Source: three-view drawing plus pictorial views. Frame: mm from the lowest corner of the part. A direction names the side the tool comes from. Coordinates: 2 decimals unless noted, no trailing zeros. Order: outer loops, then holes, each group sorted by start corner. A loop starts at its lowest first (then second) coordinate and runs counter-clockwise, first axis right, second up. Notation, with made-up numbers: (81.5, 0) - (122.5, 0) arc R23 cw to (122.5, 35) - close; hole circle Ø3 at (32, -36). An arc over 180 degrees is marked (long way). One line per question, with ' | ' between items.
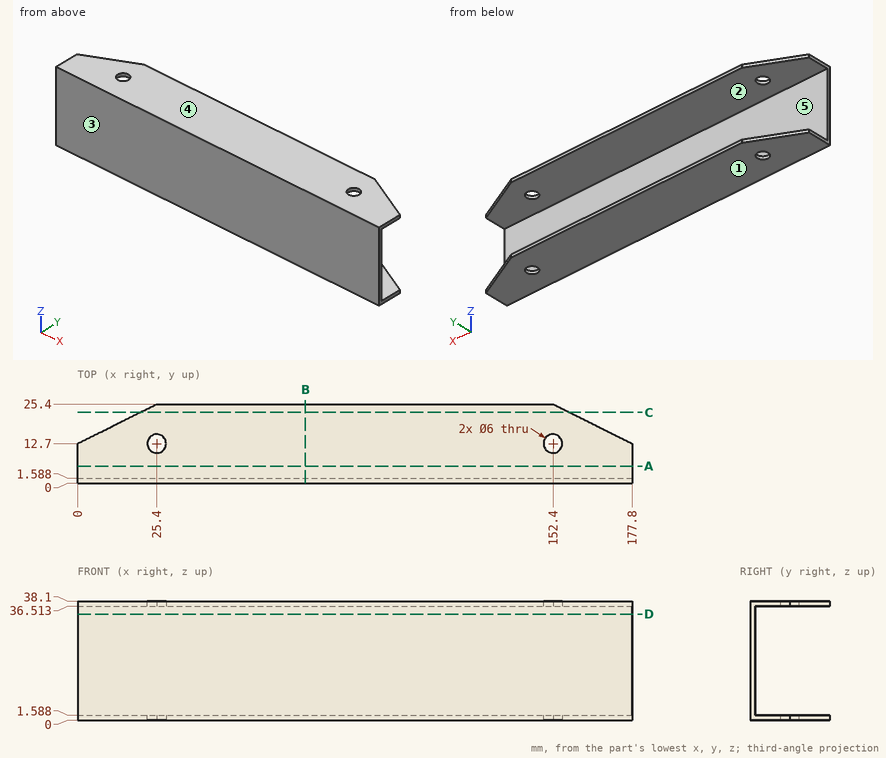
Item 1: Section C-C on y = 22.75. Return the cut outline in (x, z).
Data:
outline: (20.1, 0) - (157.7, 0) - (157.7, 1.59) - (20.1, 1.59) - close; (20.1, 36.51) - (157.7, 36.51) - (157.7, 38.1) - (20.1, 38.1) - close
Item 2: Section A-A on y = 5.5. Return the cut outline in (x, z).
Data:
outline: (0, 0) - (177.8, 0) - (177.8, 1.59) - (0, 1.59) - close; (0, 36.51) - (177.8, 36.51) - (177.8, 38.1) - (0, 38.1) - close
Item 3: Draft query along Z for the marked faces 1, 2 and 3. Return one class per face: released by +Z, released by -Z, zero draft, split by the parting line, or undercut.
Data:
face 1: released by -Z | face 2: undercut | face 3: zero draft
Item 4: Ray query, line 1 (Z direction, x = 79, y = 24); line 2 (Y direction, x = 152.4, z = 37.3); line 3 (Y direction, x = 153, z = 4.5). Return the intervals inside material, ascending.
Data:
line 1: 0 to 1.59, 36.51 to 38.1 | line 2: 0 to 9.7, 15.7 to 25.4 | line 3: 0 to 1.59
Item 5: Contact query for flat-ended pins moving along their axis: P1, Ø3.5, axis at x = 25.4, y = 12.7, coming from the -Z side; P2, Ø17.5, axis at x = 56, z = 27, coming from the +Y side. Output: stop coordinate, or through.
Data:
P1: through | P2: y = 1.59
Item 6: Section D-D on z = 34. Return the cut outline in (x, y).
Data:
outline: (0, 0) - (177.8, 0) - (177.8, 1.59) - (0, 1.59) - close
Item 7: Access query for the marked faces 4 and 5. Directions: +Z, -Z, +X, -X, +Y, -Y. A direction counts if a zero-diameter tool reaches every point of the face in a straight line with its end or side. Return the directions, or none.
Data:
face 4: +Z, +X, -X, +Y, -Y | face 5: +X, -X, +Y
Item 8: Section B-B on x = 73. Return the cut outline in (y, z).
Data:
outline: (0, 0) - (25.4, 0) - (25.4, 1.59) - (1.59, 1.59) - (1.59, 36.51) - (25.4, 36.51) - (25.4, 38.1) - (0, 38.1) - close
